Verification items for the finished model (mm, model axes). A direction names the side the tool comes from. Coordinates: 2 decimals unless noted, no trailing zeros. Order: outer loops, then holes, each group sorted by start corner. A loop starts at its lowest first (then second) coordinate and runs counter-clockwise, first axis right, second up. Notation, with made-up numbers: (20.5, 65.5) -> (40.5, 65.5) arc R12 ccw to (40.5, 84.5) -> close; hole circle Ø7 at (30, 4.25). An arc over 180 degrees is marked (long way). Write item = value, one per line. Start each with the question number.
from build123d import *

# Parameters (mm, degrees)
F1_DEPTH = 6
F3_DEPTH = 6
F4_W     = 25
F4_H     = 12
F4_H_2   = 18
F5_DEPTH = 6
F6_D     = 13


with BuildPart() as f1:
    # F0 (on Front) → F1 (new body)
    with BuildSketch(Plane.XZ):
        with BuildLine():
            Line((36.0888135582, -12.9309209585), (36.0888135582, 12.0690790415))
            Line((36.0888135582, 12.0690790415), (-27.9111864418, 12.0690790415))
            Line((-27.9111864418, 12.0690790415), (-27.9111864418, 6.5))
            Line((-27.9111864418, 6.5), (-7.9111864418, 6.5))
            Line((-7.9111864418, 6.5), (-7.9111864418, 5.9503926081))
            ThreePointArc((-7.9111864418, 5.9503926081), (-3.7036234779, 4.2075629639), (-1.9607938337, 0))
            ThreePointArc((-1.9607938337, 0), (-3.7036234779, -4.2075629639), (-7.9111864418, -5.9503926081))
            Line((-7.9111864418, -5.9503926081), (-7.9111864418, -6.5))
            Line((-7.9111864418, -6.5), (-27.9111864418, -6.5))
            Line((-27.9111864418, -6.5), (-27.9111864418, -12.9309209585))
            Line((-27.9111864418, -12.9309209585), (36.0888135582, -12.9309209585))
        make_face()
    extrude(amount=F1_DEPTH)

    # F2 (on face) → F3 (join)
    with BuildSketch(Plane.YZ.offset(36.0888135582)):
        with BuildLine():
            Line((0, -12.9309209585), (0, 12.0690790415))
            Line((0, 12.0690790415), (-18, 12.0690790415))
            ThreePointArc((-18, 12.0690790415), (-9.1611652352, 8.4079138063), (-5.5, -0.4309209585))
            ThreePointArc((-5.5, -0.4309209585), (-9.1611652352, -9.2697557234), (-18, -12.9309209585))
            Line((-18, -12.9309209585), (0, -12.9309209585))
        make_face()
        with BuildLine():
            ThreePointArc((-5.5, -0.4309209585), (-9.1611652352, 8.4079138063), (-18, 12.0690790415))
            Line((-18, 12.0690790415), (-18, 5.8190790415))
            ThreePointArc((-18, 5.8190790415), (-13.5805826176, 3.9884964239), (-11.75, -0.4309209585))
            ThreePointArc((-11.75, -0.4309209585), (-13.5805826176, -4.8503383409), (-18, -6.6809209585))
            Line((-18, -6.6809209585), (-18, -12.9309209585))
            ThreePointArc((-18, -12.9309209585), (-9.1611652352, -9.2697557234), (-5.5, -0.4309209585))
        make_face()
        with BuildLine():
            Line((-18, 5.8190790415), (-18, 12.0690790415))
            ThreePointArc((-18, 12.0690790415), (-30.5, -0.4309209585), (-18, -12.9309209585))
            Line((-18, -12.9309209585), (-18, -6.6809209585))
            ThreePointArc((-18, -6.6809209585), (-24.25, -0.4309209585), (-18, 5.8190790415))
        make_face()
    extrude(amount=-F3_DEPTH)

    # F4 (on face) → F5 (join)
    with BuildSketch(Plane(origin=(0, 0, -12.9309209585), x_dir=(1, 0, 0), z_dir=(0, 0, -1))):
        with Locations((23.5888135582, -6)):
            Rectangle(F4_W, F4_H)
        with Locations((23.5888135582, -3)):
            Rectangle(F4_W, F4_H_2)
        with BuildLine():
            ThreePointArc((11.0888135582, -12), (23.5888135582, -24.5), (36.0888135582, -12))
            Line((36.0888135582, -12), (11.0888135582, -12))
        make_face()
    extrude(amount=-F5_DEPTH)

    # F6 (through all)
    with Locations(Plane(origin=(0, 0, -12.9309209585), x_dir=(1, 0, 0), z_dir=(0, 0, -1))):
        with Locations((23.5888135582, -12)):
            Hole(F6_D / 2)


solid = f1.part
Item 1: Section check A-A (x = -10.5). Record the boundary of the cut face in (y, z), then the cut area to 3 significant figures.
Item 2: Section check D-D (y = -1.5). Record the boundary of the cut face in (x, z).
Item 3: Thickness scan on line 1 (X direction, y = -12.5, z = -6.25); line 2 (Y direction, x = 28, z = 3.25); line 3 (Z direction, x = 15.5, y = 12). Record the ranges inside material, lowest first.
Item 4: Tool access check on faces 5 (the flat face through (11, 0, 0)), 6 (the flat face through (29, 7, -6.931)), 7 (the flat face through (7, -6, 0)), 8 (the flat face through (-18, -3, 6.5)), 9 (the flat face through (11.089, 6, -10)). Record the directions out of +Z, -Z, +X, -X, +Y, -Y that give a thin tool (end or side, any length) a straight path to the whole face; none if there is none.
Item 5: Mould release check, pull along Z, two halves, no side actions. Record for faces 1 (the cylindrical face through (33.131, -30.497, -0.156)), 2 (the flat face through (-18, -3, -6.5)), 3 (the flat face through (30.089, -10, 0)), 4 (the flat face through (16, 2, -12.931)): pulls with the +Z half, pulls with the -Z half, needs draft (parallel to the pull), parting line crosses it, or undercut.
Item 6: Gauge pin test, flat ends, axial feed: P1, Ø12.5, axis at x = 9.5, z = 4.5, coming from the -Y side; P2, Ø10, axis at y = 17.5, z = -9, coming from the -X side; P3, Ø7.5, axis at x = 26, y = 16, coming from the +Z side. Record the tip position at first contact, or that the pin passes through.
Item 7: Section check C-C (z = -1.25). Record the boundary of the cut face in (x, y), then the cut area to 3 significant figures.
Item 8: Section check B-B (y = -21.5). Record the boundary of the cut face in (x, z).
Filled sheet:
q1.outline = (-6, -12.93) -> (0, -12.93) -> (0, -6.5) -> (-6, -6.5) -> close; (-6, 6.5) -> (0, 6.5) -> (0, 12.07) -> (-6, 12.07) -> close
q1.area = 72.0 mm^2
q2.outline = (-27.91, -12.93) -> (36.09, -12.93) -> (36.09, 12.07) -> (-27.91, 12.07) -> (-27.91, 6.5) -> (-7.91, 6.5) -> (-7.91, 5.95) arc R5.95 cw to (-7.91, -5.95) -> (-7.91, -6.5) -> (-27.91, -6.5) -> close
q3.line_1 = 30.09 to 36.09
q3.line_2 = -6 to 0
q3.line_3 = -12.93 to -6.93
q4.face_5 = +Z, -X, +Y
q4.face_6 = +Z, +X, -X, +Y
q4.face_7 = +Z, -Z, -X, -Y
q4.face_8 = -X, +Y, -Y
q4.face_9 = +Z, -Z, -X, +Y
q5.face_1 = parting line crosses it
q5.face_2 = undercut
q5.face_3 = needs draft
q5.face_4 = pulls with the -Z half
q6.P1 = -6
q6.P2 = 11.1
q6.P3 = -6.93
q7.outline = (-2.09, -6) -> (30.09, -6) -> (30.09, -11.8) -> (36.09, -11.8) -> (36.09, 0) -> (-2.09, 0) -> close; (30.09, -30.47) -> (36.09, -30.47) -> (36.09, -24.2) -> (30.09, -24.2) -> close
q7.area = 302 mm^2
q8.outline = (30.09, -12.43) -> (36.09, -12.43) -> (36.09, -5.61) -> (30.09, -5.61) -> close; (30.09, 4.75) -> (36.09, 4.75) -> (36.09, 11.57) -> (30.09, 11.57) -> close
